```python
from build123d import *

# Parameters (mm, degrees)
BOSS_EXTRUDE1_DEPTH     = 1270
SKETCH1_5_W             = 762
SKETCH1_5_H             = 254
BOSS_EXTRUDE2_DEPTH     = 508
BOSS_EXTRUDE3_DEPTH     = 254
SKETCH1_7_W             = 254
SKETCH1_7_H             = 508
BOSS_EXTRUDE4_DEPTH     = 1270
CUT_EXTRUDE1_DEPTH      = 254
CUT_EXTRUDE1_DEPTH_BACK = 255


with BuildPart() as part:
    # Sketch1 → Boss-Extrude1 (new body)
    with BuildSketch(Plane.XY):
        Polygon((0, 254), (0, 0), (762, 0), (762, 254), (254, 254), align=None)
    extrude(amount=BOSS_EXTRUDE1_DEPTH)

    # Sketch1<5> → Boss-Extrude2 (add)
    with BuildSketch(Plane.XY):
        with Locations((1143, 127)):
            Rectangle(SKETCH1_5_W, SKETCH1_5_H)
    extrude(amount=BOSS_EXTRUDE2_DEPTH)

    # Sketch1<6> → Boss-Extrude3 (add)
    with BuildSketch(Plane.XY):
        with BuildLine():
            Line((254, 762), (254, 254))
            Line((254, 254), (762, 254))
            Line((762, 254), (1524, 254))
            Line((1524, 254), (1524, 1015.999999044))
            ThreePointArc((1524, 1015.999999044), (1449.605122957, 1195.605122281), (1270, 1270))
            Line((1270, 1270), (1270, 508))
            Line((1270, 508), (508, 508))
            Line((508, 508), (508, 762))
            Line((508, 762), (254, 762))
        make_face()
    extrude(amount=BOSS_EXTRUDE3_DEPTH)

    # Sketch1<7> → Boss-Extrude4 (add)
    with BuildSketch(Plane.XY):
        with Locations((127, 508)):
            Rectangle(SKETCH1_7_W, SKETCH1_7_H)
    extrude(amount=BOSS_EXTRUDE4_DEPTH)

    # Sketch2 → Cut-Extrude1 (cut, two sides)
    with BuildSketch(Plane(origin=(254, 0, 0), x_dir=(0, 0, -1), z_dir=(1, 0, 0))) as cut_extrude1_sk:
        Polygon((2664.325511968, 2221.162755984), (-254, 762), (-1270, 254), (-4188.325511968, -1205.162755984), (-7106.651023936, 4631.488267952), (-254, 8057.813779919), align=None)
    extrude(amount=CUT_EXTRUDE1_DEPTH, mode=Mode.SUBTRACT)
    extrude(cut_extrude1_sk.sketch, amount=-CUT_EXTRUDE1_DEPTH_BACK, mode=Mode.SUBTRACT)


solid = part.part
```
For this review, take the finished solid that the model builds, in its own axes (mm). A direction names the side the tool comes from. Coordinates: 2 decimals unless noted, no trailing zeros. Write each loop counter-clockwise with the first axis right and the second up, starting at its lowest first coordinate (ties: lowest second). Pieces come first, ordered by that corner, then holes. Notation, with made-up numbers: (-13, -8.75) -> (30, -8.75) arc R19 cw to (30, 11.25) -> close; hole circle Ø10 at (-13.75, 9.25). An arc over 180 degrees is marked (long way). Put each result on its own line as item: value.
Q1. Wall thickness on L1, parallel to Y at x = 637.5, z = 922.5; L2, parallel to Y at x = 1145, z = 110: over which ranges is each line inside the solid? List them lowest first.
From the geometry:
L1: y = 0 to 254
L2: y = 0 to 508
Q2. Take a section at A-A, the plane y = 608.5. State the section outline as (x, z) points.
From the geometry:
outline: (0, 0) -> (508, 0) -> (508, 254) -> (254, 254) -> (254, 561) -> (0, 561) -> close; (1270, 0) -> (1524, 0) -> (1524, 254) -> (1270, 254) -> close
Q3. Take a section at C-C, the plane z = 773.5. State the section outline as (x, y) points, then the cut area to 3 significant figures.
From the geometry:
outline: (0, 0) -> (762, 0) -> (762, 254) -> (254, 254) -> (254, 502.25) -> (0, 502.25) -> close
area: 257,000 mm2
Q4. The part is to be moulded in two halves that separate along X. For faces 4 (the flat face through (508, 633, 125)), 5 (the flat face through (762, 125, 884)), 6 (the flat face through (894, 508, 125)), 7 (the flat face through (1021, 430, 254)), say which applies: +X half, -X half, draft (parallel to the pull), parting line (faces both ways), or undercut.
From the geometry:
face 4: undercut
face 5: +X half
face 6: undercut
face 7: draft
Q5. Take a section at D-D, the plane y = 974.5. State the section outline as (x, z) points, then the cut area to 3 significant figures.
From the geometry:
outline: (1270, 0) -> (1524, 0) -> (1524, 254) -> (1270, 254) -> close
area: 64,500 mm2
Q6. Tool access review of faces 1 (the flat face through (1138, 129, 508)), 2 (the flat face through (254, 448, 642)), 3 (the flat face through (1270, 894, 125)): name each direction out of +Z, -Z, +X, -X, +Y, -Y from which nothing blocks a thin tool from reaching the whole face with its end or side.
From the geometry:
face 1: +Z, +X, +Y, -Y
face 2: +Z, +X, +Y
face 3: +Z, -Z, +Y
Q7. Take a section at B-B, the plane x = 692. State the section outline as (y, z) points.
From the geometry:
outline: (0, 0) -> (508, 0) -> (508, 254) -> (254, 254) -> (254, 1270) -> (0, 1270) -> close
Q8. Clearance check with flat-ended pins moving along their axes: pin 1 Ø5 at (x, z) = (677, 892.5) entering from +Y; pin 2 Ø5 at (x, y) = (346, 726.5) entering from +Z. State where each tip first meets the part, or that it passes through.
From the geometry:
pin 1: stops at y = 254
pin 2: stops at z = 254
